Verification items for the finished model (mm, model axes). Face numbers are marked on the shaded views. A direction names the side the tool comes from. Round coordinates to 2 decimals unless told otherwise and drop trailing zeros. Loops run counter-clockwise (first coordinate to the right, second up) from the corner with the lowest first, then second, coordinate; pieces in that order, holes last. Notation, with made-up numbers: M 14.25,10.5 L 73.25,10.5 A27 ccw 73.25,32.5 Z; hole C -14.5,3 d10. An arc over 180 degrees is marked long. Answer as CSV lines item,"result".
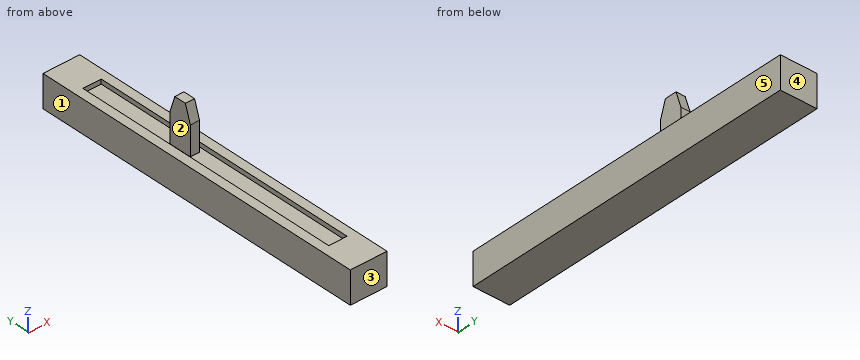
```python
from build123d import *

# Parameters (mm, degrees)
SKETCH1_W           = 8
SKETCH1_H           = 75
BOSS_EXTRUDE1_DEPTH = 7
SKETCH2_W           = 4
SKETCH2_H           = 60
CUT_EXTRUDE1_DEPTH  = 1
BOSS_EXTRUDE2_DEPTH = 1


with BuildPart() as part:
    # Sketch1 → Boss-Extrude1 (new body)
    with BuildSketch(Plane.XY):
        Rectangle(SKETCH1_W, SKETCH1_H)
    extrude(amount=BOSS_EXTRUDE1_DEPTH)

    # Sketch2 → Cut-Extrude1 (cut)
    with BuildSketch(Plane.XY.offset(7)):
        Rectangle(SKETCH2_W, SKETCH2_H)
    extrude(amount=-CUT_EXTRUDE1_DEPTH, mode=Mode.SUBTRACT)

    # Sketch3 → Boss-Extrude2 (add, symmetric)
    with BuildSketch(Plane(origin=(0, 0, 0), x_dir=(0, 0, -1), z_dir=(1, 0, 0))):
        Polygon((-5.362926248, 9.895130651), (-12.32555201, 9.895130651), (-16, 8.689278514), (-16, 6.100982787), (-12.32555201, 4.895130651), (-5.362926248, 4.895130651), align=None)
    extrude(amount=BOSS_EXTRUDE2_DEPTH, both=True)


solid = part.part
```
1) Section check A-A (x = 0.25). Record the cut outline in (y, z), plus the area to 3 significant figures.
Here are the results:
outline,"M -37.5,0 L 37.5,0 L 37.5,7 L 30,7 L 30,6 L 9.9,6 L 9.9,12.33 L 8.69,16 L 6.1,16 L 4.9,12.33 L 4.9,6 L -30,6 L -30,7 L -37.5,7 Z"
area,"511 mm^2"
2) Draft check along Y on the marked faces 3, 4 and 5. Enter one of: +Y half, -Y half, draft (parallel to the pull), parting line (faces both ways), or undercut.
Here are the results:
face 3,"-Y half"
face 4,"+Y half"
face 5,"draft"
3) Go/stop test with flat-tipped pins: pin 1 (3 mm diameter, centred on x = 1, z = 11.5, fed in from -Y); pin 2 (6 mm diameter, centred on y = -1, z = 13, fed in from -X); pin 3 (5.5 mm diameter, centred on y = 6.5, z = 11.5, fed in from +X); pin 4 (4.5 mm diameter, centred on x = -0.5, y = -7, fed in from +Z). Record where each tip stops, or that it passes through.
Here are the results:
pin 1,"stops at y = 4.9"
pin 2,"passes through"
pin 3,"stops at x = 1"
pin 4,"stops at z = 7"
4) Material ranges on probe 1 along Z at (x, y) = (0, -10); probe 2 along Z at (x, y) = (-3, -4); probe 3 along Y at (x, z) = (-0.25, 9.5), recorded low to high.
Here are the results:
probe 1,"z = 0 to 6"
probe 2,"z = 0 to 7"
probe 3,"y = 4.9 to 9.9"
5) Set-up check for the marked faces 1 and 2: record each of +Z, -Z, +X, -X, +Y, -Y from which the full face is reachable in a straight line by a thin tool's end or side.
Here are the results:
face 1,"+Z, -Z, -X, +Y, -Y"
face 2,"+Z"
6) Section check C-C (z = 9). Record the cut outline in (x, y), plus the area to 3 significant figures.
Here are the results:
outline,"M -1,4.9 L 1,4.9 L 1,9.9 L -1,9.9 Z"
area,"10.0 mm^2"
7) Section check D-D (z = 13.75). Record the cut outline in (x, y), plus the area to 3 significant figures.
Here are the results:
outline,"M -1,5.36 L 1,5.36 L 1,9.43 L -1,9.43 Z"
area,"8.13 mm^2"
8) Section check B-B (y = 25.5). Record the cut outline in (x, z).
Here are the results:
outline,"M -4,0 L 4,0 L 4,7 L 2,7 L 2,6 L -2,6 L -2,7 L -4,7 Z"
